Part print with two shaded views. Sizes in mm from the minimum x, y, z corner. A direction names the side the tool comes from. Give positions to 0.01 mm unless a question says otherwise; leave off trailing zeros. Order: outer loops, then holes, each group sorted by start corner. A loop starts at its lowest first (then second) coordinate and runs counter-clockwise, first axis right, second up. Notation, with made-up numbers: (-12, -23.5) -> (41, -23.5) arc R22 ccw to (41, 13.5) -> close; hole circle Ø10 at (-33.5, 24). An arc over 180 degrees is marked (long way). Answer as CSV lines item,"result".
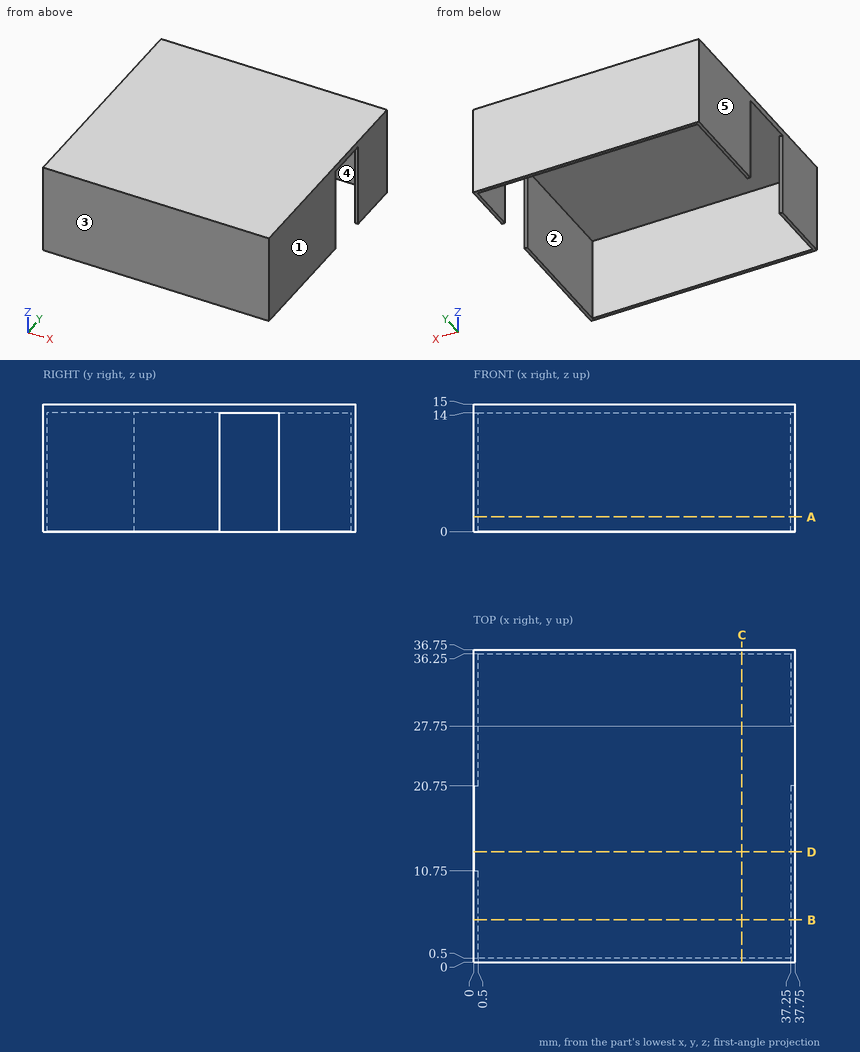
1) Band-saw the part on D-D, the plane y = 13. Write the cut outline in (x, z), then the cut area to 4 significant figures.
Data:
outline,"(0, 14) -> (37.25, 14) -> (37.25, 0) -> (37.75, 0) -> (37.75, 15) -> (0, 15) -> close"
area,"44.75 mm2"
2) Pull direction Y, two halves, no side cores. Call the marked faces 3, 4 and 5: pulls with the +Y half, pulls with the -Y half, needs draft (parallel to the pull), parting line crosses it, or undercut.
Data:
face 3,"pulls with the -Y half"
face 4,"undercut"
face 5,"needs draft"
3) Pin check, flat tips, straight feed: P1, Ø2, axis at x = 33, y = 7.5, coming from the -Z side; P2, Ø4, axis at y = 25, z = 9.5, coming from the +X side. Stop position of each tip, or through.
Data:
P1,"stops at z = 14"
P2,"stops at x = 0.5"
4) Wall check: line 1 along Y through (x, z) = (4, 9.5); line 2 along X through (y, z) = (35.5, 5.75); line 3 along Z through (x, y) = (33.5, 34). Give the ranges that are in metal, low to high. Write a range as [from, to].
Data:
line 1,"y = [0, 0.5], [36.25, 36.75]"
line 2,"x = [0, 0.5], [37.25, 37.75]"
line 3,"z = [14, 15]"
5) Band-saw the part on A-A, the plane z = 1.75. Write the cut outline in (x, y), then the cut area to 3 significant figures.
Data:
outline,"(0, 0) -> (37.75, 0) -> (37.75, 20.75) -> (37.25, 20.75) -> (37.25, 0.5) -> (0.5, 0.5) -> (0.5, 10.75) -> (0, 10.75) -> close; (0, 20.75) -> (0.5, 20.75) -> (0.5, 36.25) -> (37.25, 36.25) -> (37.25, 27.75) -> (37.75, 27.75) -> (37.75, 36.75) -> (0, 36.75) -> close"
area,"65.0 mm2"
6) Which spindle directions (+Z, -Z, +X, -X, +Y, -Y) get a long thin tool onto all of the face, cutting with end or side? Do the marked faces 1 and 2. Say none if no direction does.
Data:
face 1,"+Z, -Z, +X, +Y, -Y"
face 2,"-Z"
7) Band-saw the part on C-C, the plane x = 31.5. Write the cut outline in (y, z), then the cut area to 4 significant figures.
Data:
outline,"(0, 0) -> (0.5, 0) -> (0.5, 14) -> (36.25, 14) -> (36.25, 0) -> (36.75, 0) -> (36.75, 15) -> (0, 15) -> close"
area,"50.75 mm2"
8) Band-saw the part on B-B, the plane y = 5. Write the cut outline in (x, z).
Data:
outline,"(0, 0) -> (0.5, 0) -> (0.5, 14) -> (37.25, 14) -> (37.25, 0) -> (37.75, 0) -> (37.75, 15) -> (0, 15) -> close"
